Can you work these out from the model? Positions are in its coordinate system, mm. A direction names the side the tool comes from. Give positions to 0.01 mm unless a question says otherwise; leave off trailing zeros. Loops run counter-clockwise (first coordinate to the right, second up) from the corner with the lowest first, then second, coordinate; pieces in that order, holes last. Notation, with made-up numbers: (85, 41) - (107, 41) arc R15 cw to (107, 67) - close; hole circle Ø3 at (10.25, 58.25). An arc over 180 degrees is marked (long way). Answer as a JSON object with one key per item and string values.
```python
from build123d import *

# Parameters (mm, degrees)
SKETCH_1_W      = 10.7
SKETCH_1_H      = 4.4
EXTRUDE_1_DEPTH = 20.3
SKETCH_2_R      = 0.25
EXTRUDE_2_DEPTH = 5
SKETCH_3_R      = 1.5
EXTRUDE_3_DEPTH = 3.5
FILLET_1_R      = 1.5


with BuildPart() as part:
    # 草图1 → 凸台-拉伸1 (new body)
    with BuildSketch(Plane.XY):
        Rectangle(SKETCH_1_W, SKETCH_1_H)
    extrude(amount=EXTRUDE_1_DEPTH)

    # 草图2 → 凸台-拉伸2 (add)
    with BuildSketch(Plane(origin=(0, 0, 0), x_dir=(-1, 0, 0), z_dir=(0, 0, -1))):
        with Locations(Location((-2.6, 1.27, 0), (0, 0, 180))):
            Circle(SKETCH_2_R)
        with Locations(Location((-0.7, 1.27, 0), (0, 0, 180))):
            Circle(SKETCH_2_R)
        with Locations(Location((1.2, 1.27, 0), (0, 0, 180))):
            Circle(SKETCH_2_R)
        with Locations(Location((3.1, 1.27, 0), (0, 0, 180))):
            Circle(SKETCH_2_R)
        with Locations(Location((3.1, -1.27, 0), (0, 0, 180))):
            Circle(SKETCH_2_R)
        with Locations(Location((1.2, -1.27, 0), (0, 0, 180))):
            Circle(SKETCH_2_R)
        with Locations(Location((-0.7, -1.27, 0), (0, 0, 180))):
            Circle(SKETCH_2_R)
        with Locations(Location((-2.6, -1.27, 0), (0, 0, 180))):
            Circle(SKETCH_2_R)
    extrude(amount=EXTRUDE_2_DEPTH)

    # 草图3 → 凸台-拉伸3 (add)
    with BuildSketch(Plane(origin=(5.35, 0, 0), x_dir=(0, 0, -1), z_dir=(1, 0, 0))):
        with Locations(Location((-2.54, 0, 0), (0, 0, 270))):
            Circle(SKETCH_3_R)
        with Locations(Location((-7.62, 0, 0), (0, 0, 270))):
            Circle(SKETCH_3_R)
        with Locations(Location((-12.7, 0, 0), (0, 0, 270))):
            Circle(SKETCH_3_R)
        with Locations(Location((-17.78, 0, 0), (0, 0, 270))):
            Circle(SKETCH_3_R)
    extrude(amount=EXTRUDE_3_DEPTH)

    # 圆角1
    fillet_1_edges = [part.edges().sort_by_distance(p)[0] for p in [
        (8.85, 1.5, 2.54),
        (8.85, 1.5, 7.62),
        (8.85, 1.5, 12.7),
        (8.85, 1.5, 17.78),
    ]]
    fillet(fillet_1_edges, radius=FILLET_1_R)


solid = part.part
```
1) Imagine slicing it at D-D on y = 0.25. Write out the boundary of the cut face in (x, z), and give its area (3 significant figures).
Check sheet entries:
{"outline": "(-5.35, 0) - (5.35, 0) - (5.35, 1.06) - (7.35, 1.06) arc R1.48 ccw to (7.35, 4.02) - (5.35, 4.02) - (5.35, 6.14) - (7.35, 6.14) arc R1.48 ccw to (7.35, 9.1) - (5.35, 9.1) - (5.35, 11.22) - (7.35, 11.22) arc R1.48 ccw to (7.35, 14.18) - (5.35, 14.18) - (5.35, 16.3) - (7.35, 16.3) arc R1.48 ccw to (7.35, 19.26) - (5.35, 19.26) - (5.35, 20.3) - (-5.35, 20.3) - close", "area": "255 mm2"}
2) I need wall thicknesses on L1, parallel to Z at x = -4.25, y = -2; L2, parallel to X at y = 1.8, z = 14.25; L3, parallel to Y at x = 8, z = 17.5. Which ranges of each line are inside material? Lowest first, please.
Check sheet entries:
{"L1": "0 to 20.3", "L2": "-5.35 to 5.35", "L3": "-1.32 to 1.32"}
3) Which directions (+Z, -Z, +X, -X, +Y, -Y) give clear straight access to the entire face, cutting with the end or side of a thin tool? Please do faces 4 (the flat face through (0, 0, 20.3)), 5 (the cylindrical face through (6.336, 0.325, 9.084)).
Check sheet entries:
{"face 4": "+Z, +X, -X, +Y, -Y", "face 5": "+X"}
4) Imagine slicing it at C-C on x = 7. Write out the boundary of the cut face in (y, z).
Check sheet entries:
{"outline": "circle Ø3 at (0, 2.54); circle Ø3 at (0, 7.62); circle Ø3 at (0, 12.7); circle Ø3 at (0, 17.78)"}
5) Imagine slicing it at A-A on z = -3. Write out the boundary of the cut face in (x, y).
Check sheet entries:
{"outline": "circle Ø0.5 at (-3.1, -1.27); circle Ø0.5 at (-3.1, 1.27); circle Ø0.5 at (-1.2, -1.27); circle Ø0.5 at (-1.2, 1.27); circle Ø0.5 at (0.7, -1.27); circle Ø0.5 at (0.7, 1.27); circle Ø0.5 at (2.6, -1.27); circle Ø0.5 at (2.6, 1.27)"}
6) If we mould it in two halves opening along Z, with no side actions, what happens to faces 1 (the cylindrical face through (6.336, 0.325, 14.164)), 2 (the flat face through (0, 0, 0)), 3 (the flat face through (-5.35, 0, 10))? For each: released by +Z, released by -Z, zero draft, split by the parting line, or undercut.
Check sheet entries:
{"face 1": "undercut", "face 2": "released by -Z", "face 3": "zero draft"}
7) Imagine slicing it at B-B on x = 0.7. Write out the boundary of the cut face in (y, z), and give its area (3 significant figures).
Check sheet entries:
{"outline": "(-2.2, 0) - (-1.52, 0) - (-1.52, -5) - (-1.02, -5) - (-1.02, 0) - (1.02, 0) - (1.02, -5) - (1.52, -5) - (1.52, 0) - (2.2, 0) - (2.2, 20.3) - (-2.2, 20.3) - close", "area": "94.3 mm2"}
8) I'm going to push a flat-ended pin straight in: P1, Ø2, axis at y = 1.5, z = 0, coming from the +X side. Where does the tip first touch, or does it pass through?
Check sheet entries:
{"P1": "x = 5.35"}
